from build123d import *

# Parameters (mm, degrees)
SKETCH1_R           = 3.5
SKETCH1_R_2         = 2.25
BOSS_EXTRUDE1_DEPTH = 3
SKETCH3_R           = 2.25
BOSS_EXTRUDE2_DEPTH = 3
FILLET1_R           = 3
FILLET2_R           = 3


with BuildPart() as part:
    # Sketch1 → Boss-Extrude1 (new body)
    with BuildSketch(Plane.XY):
        Polygon((120, 29.7), (96, 29.7), (96, -29.7), (120, -29.7), (120, -42.45), (0, -42.45), (0, 42.45), (120, 42.45), align=None)
        with Locations((5, 36.2)):
            Circle(SKETCH1_R, mode=Mode.SUBTRACT)
        with Locations((75, 36.2)):
            Circle(SKETCH1_R, mode=Mode.SUBTRACT)
        with Locations((5, -36.2)):
            Circle(SKETCH1_R, mode=Mode.SUBTRACT)
        with Locations((75, -36.2)):
            Circle(SKETCH1_R, mode=Mode.SUBTRACT)
        with Locations((116, 36.2)):
            Circle(SKETCH1_R_2, mode=Mode.SUBTRACT)
        with Locations((101, 36.2)):
            Circle(SKETCH1_R_2, mode=Mode.SUBTRACT)
        with Locations((101, -36.2)):
            Circle(SKETCH1_R_2, mode=Mode.SUBTRACT)
        with Locations((116, -36.2)):
            Circle(SKETCH1_R_2, mode=Mode.SUBTRACT)
    extrude(amount=-BOSS_EXTRUDE1_DEPTH)

    # Sketch3 → Boss-Extrude2 (add)
    with BuildSketch(Plane(origin=(96, 0, 0), x_dir=(0, 0, -1), z_dir=(1, 0, 0))):
        with BuildLine():
            Line((0, 29.7), (0, -29.7))
            Line((0, -29.7), (3, -29.7))
            Line((3, -29.7), (3, -25))
            ThreePointArc((3, -25), (4.730773609, -20.207711731), (9.124273828, -17.627254412))
            Line((9.124273828, -17.627254412), (50, -10))
            Line((50, -10), (50, 10))
            Line((50, 10), (9.124273828, 17.627254412))
            ThreePointArc((9.124273828, 17.627254412), (4.730773609, 20.207711731), (3, 25))
            Line((3, 25), (3, 29.7))
            Line((3, 29.7), (0, 29.7))
        make_face()
        with Locations((29, 0)):
            Circle(SKETCH3_R, mode=Mode.SUBTRACT)
        with Locations((44, 0)):
            Circle(SKETCH3_R, mode=Mode.SUBTRACT)
        with BuildLine():
            Line((9.600816641, 14.566475289), (34.500680534, 9.476605143))
            ThreePointArc((34.500680534, 9.476605143), (36.458725143, 6.574848986), (33.596044735, 4.560106232))
            Line((33.596044735, 4.560106232), (8.515253682, 8.666676596))
            ThreePointArc((8.515253682, 8.666676596), (6.049529828, 12.170140924), (9.600816641, 14.566475289))
        make_face(mode=Mode.SUBTRACT)
        with BuildLine():
            ThreePointArc((33.596044735, -4.560106232), (36.458725143, -6.574848986), (34.500680534, -9.476605143))
            Line((34.500680534, -9.476605143), (9.600816641, -14.566475289))
            ThreePointArc((9.600816641, -14.566475289), (6.049529828, -12.170140924), (8.515253682, -8.666676596))
            Line((8.515253682, -8.666676596), (33.596044735, -4.560106232))
        make_face(mode=Mode.SUBTRACT)
    extrude(amount=BOSS_EXTRUDE2_DEPTH)

    # Fillet1
    fillet1_edges = [part.edges().sort_by_distance(p)[0] for p in [
        (99, 0, 0),
    ]]
    fillet(fillet1_edges, radius=FILLET1_R - 0.0001)  # a hair under: the kernel refuses the full size

    # Fillet2
    fillet2_edges = [part.edges().sort_by_distance(p)[0] for p in [
        (96, 0, -3),
    ]]
    fillet(fillet2_edges, radius=FILLET2_R - 0.0001)  # a hair under: the kernel refuses the full size


solid = part.part
Design review of the part built by this model. Coordinates are the model's own, in mm. A direction names the side the tool comes from. Give positions to 0.01 mm unless a question says otherwise; leave off trailing zeros. Write each loop counter-clockwise with the first axis right and the second up, starting at its lowest first coordinate (ties: lowest second). Pieces come first, ordered by that corner, then holes. Notation, with made-up numbers: M 43,-6 L 54,-6 A28 cw 54,32 Z; hole C 69,37 d7. An arc over 180 degrees is marked long. Answer as a JSON object with one key per item and string values. Group by question number.
1) We need section A-A (y = 0). Give the boundary of the cut face in (x, z).
2) Clearance check with flat-ended pins moving along their axes: pin 1 Ø4 at (x, y) = (5, -36.2) entering from -Z; pin 2 Ø8 at (x, y) = (100.5, -13) entering from +Z; pin 3 Ø14 at (y, z) = (3.5, -28.5) entering from +X; pin 4 Ø3 at (x, y) = (22.5, -3) entering from -Z. State where each tip first meets the part, or that it passes through.
3) We need section D-D (z = -44). Give the boundary of the cut face in (x, y), and give its area (3 significant figures).
4) For line 1 along X through (y, z) = (-36, -2); line 2 along Y through (x, z) = (116, -1.65); line 3 along Z through (x, y) = (64, -4.5), list the stretches that pass through material, from the lowest coordinate up.
5) Mouldability with a two-part tool opening along X and no side actions: class faces 4 (the face through (120, 36, -1)), 5 (the face through (96, -4, -28)), 6 (the face through (103.08, -37.06, -1.48)), 7 (the face through (76.615, -39.305, -1.479)) as released by +X, released by -X, zero draft, split by the parting line, or undercut.
6) Tool access review of faces 1 (the face through (98.1, -0.42, -0.86)), 2 (the face through (97.479, 12.057, -21.876)), 3 (the face through (6.615, -39.305, -1.479)): name each direction out of +Z, -Z, +X, -X, +Y, -Y from which nothing blocks a thin tool from reaching the whole face with its end or side.
7) We need section C-C (y = -36.2). Give the boundary of the cut face in (x, z).
8) We need section B-B (x = 5). Give the boundary of the cut face in (y, z).
Answer key:
{
 "1": {"outline": "M 0,-3 L 93,-3 A3 cw 96,-6 L 96,-26.75 L 99,-26.75 L 99,-3 A3 ccw 96,0 L 0,0 Z; M 96,-50 L 99,-50 L 99,-46.25 L 96,-46.25 Z; M 96,-41.75 L 99,-41.75 L 99,-31.25 L 96,-31.25 Z"},
 "2": {"pin 1": "passes through", "pin 2": "stops at z = -0.04", "pin 3": "stops at x = 99", "pin 4": "stops at z = -3"},
 "3": {"outline": "M 96,-11.12 L 99,-11.12 L 99,-2.25 L 96,-2.25 Z; M 96,2.25 L 99,2.25 L 99,11.12 L 96,11.12 Z", "area": "53.2 mm²"},
 "4": {"line 1": "x = 0 to 1.51, 8.49 to 71.51, 78.49 to 98.76, 103.24 to 113.76, 118.24 to 120", "line 2": "y = -42.45 to -38.45, -33.95 to -29.7, 29.7 to 33.95, 38.45 to 42.45", "line 3": "z = -3 to 0"},
 "5": {"face 4": "released by +X", "face 5": "released by -X", "face 6": "undercut", "face 7": "undercut"},
 "6": {"face 1": "+Z, +X", "face 2": "+X, -X", "face 3": "+Z, -Z"},
 "7": {"outline": "M 0,-3 L 1.5,-3 L 1.5,0 L 0,0 Z; M 8.5,-3 L 71.5,-3 L 71.5,0 L 8.5,0 Z; M 78.5,-3 L 98.75,-3 L 98.75,0 L 78.5,0 Z; M 103.25,-3 L 113.75,-3 L 113.75,0 L 103.25,0 Z; M 118.25,-3 L 120,-3 L 120,0 L 118.25,0 Z"},
 "8": {"outline": "M -42.45,-3 L -39.7,-3 L -39.7,0 L -42.45,0 Z; M -32.7,-3 L 32.7,-3 L 32.7,0 L -32.7,0 Z; M 39.7,-3 L 42.45,-3 L 42.45,0 L 39.7,0 Z"}
}
